The listing builds one solid part. Answer for the finished solid, in the listing's coordinates (mm). Face numbers are marked on the shaded views. A direction names the side the tool comes from. Round coordinates to 2 decimals unless told otherwise and drop trailing zeros. Write each loop counter-clockwise with the first axis right and the second up, starting at its lowest first coordinate (ties: lowest second). Pieces come first, ordered by that corner, then holes. Notation, with made-up numbers: (63.25, 79.5) - (103.25, 79.5) arc R16 cw to (103.25, 88.5) - close; hole circle Ø2 at (-17.5, 76.5). An arc over 180 degrees is marked (long way). Answer in a Markdown table with one row per item.
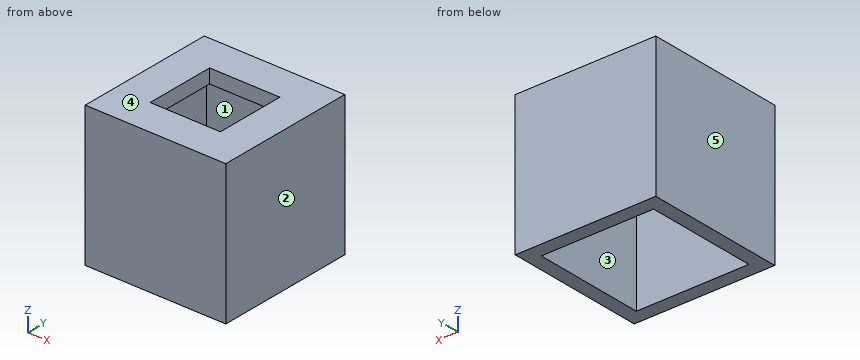
Autodesk Inventor part; units mm, degrees
ref_plane "YZ Plane" through (0, 0, 0) normal (1, 0, 0) x (0, 1, 0)
ref_plane "XZ Plane" through (0, 0, 0) normal (0, 1, 0) x (-1, 0, 0)
ref_plane "XY Plane" through (0, 0, 0) normal (0, 0, 1) x (1, 0, 0)
sketch "Sketch1" plane through (0, 0, 0) normal (0, 0, 1) x (1, 0, 0)
  line L0 (-24.3417, 44.0972) -> (51.8583, 44.0972)
  line L1 (51.8583, 44.0972) -> (51.8583, -32.1028)
  line L2 (51.8583, -32.1028) -> (-24.3417, -32.1028)
  line L3 (-24.3417, -32.1028) -> (-24.3417, 44.0972)
  point P0 (0, 0)
  dimension "d0" = 76.2
  dimension "d1" = 76.2
extrude "Extrusion1" add sketch "Sketch1" along normal blind 76.2
shell "Shell1" thickness 7.62 removed faces 1 at (1.0583, 18.6972, 0)
sketch "Sketch2" plane through (0, 0, 76.2) normal (0, 0, 1) x (1, 0, 0)
  line L0 (-5.2917, 25.0472) -> (32.8083, 25.0472)
  line L1 (32.8083, 25.0472) -> (32.8083, -13.0528)
  line L2 (32.8083, -13.0528) -> (-5.2917, -13.0528)
  line L3 (-5.2917, -13.0528) -> (-5.2917, 25.0472)
  line L4 (51.8583, 44.0972) -> (-24.3417, 44.0972)
  line L5 (51.8583, -32.1028) -> (51.8583, 44.0972)
  point P0 (0, 0)
  dimension "d5" = 38.1
  dimension "d6" = 38.1
  dimension "d7" = 19.05
  dimension "d8" = 19.05
extrude "Extrusion2" cut sketch "Sketch2" against normal blind 25.4
properties part number "secondary_part"
(1) Section C-C (y = 4) is taken. Give the vertices of the cut face in (x, z).
Checked values:
| item | result |
|---|---|
| outline | (-24.34, 0) - (-16.72, 0) - (-16.72, 68.58) - (-5.29, 68.58) - (-5.29, 76.2) - (-24.34, 76.2) - close; (32.81, 68.58) - (44.24, 68.58) - (44.24, 0) - (51.86, 0) - (51.86, 76.2) - (32.81, 76.2) - close |
(2) For the marked faces 1 and 2, determine the directions among +Z, -Z, +X, -X, +Y, -Y from which every point of the face is accessible in a straight line to the end or side of a thin tool.
Checked values:
| item | result |
|---|---|
| face 1 | -Z |
| face 2 | +Z, -Z, +X, +Y, -Y |
(3) Section A-A (z = 23) is taken. Give the vertices of the cut face in (x, y), and give its area (3 significant figures).
Checked values:
| item | result |
|---|---|
| outline | (-24.34, -32.1) - (51.86, -32.1) - (51.86, 44.1) - (-24.34, 44.1) - close; hole (-16.72, -24.48) - (44.24, -24.48) - (44.24, 36.48) - (-16.72, 36.48) - close |
| area | 2,090 mm2 |
(4) For a pull along X with two mould halves and no side action, classify the marked faces 3, 4 and 5 as pulls with the +X half, pulls with the -X half, needs draft (parallel to the pull), parting line crosses it, or undercut.
Checked values:
| item | result |
|---|---|
| face 3 | undercut |
| face 4 | needs draft |
| face 5 | pulls with the -X half |
(5) Section B-B (x = 0) is taken. Give the vertices of the cut face in (y, z).
Checked values:
| item | result |
|---|---|
| outline | (-32.1, 0) - (-24.48, 0) - (-24.48, 68.58) - (-13.05, 68.58) - (-13.05, 76.2) - (-32.1, 76.2) - close; (25.05, 68.58) - (36.48, 68.58) - (36.48, 0) - (44.1, 0) - (44.1, 76.2) - (25.05, 76.2) - close |
(6) Find the intervals of material crossed by line 1 (X direction, y = 15.5, z = 35.5); line 2 (Y direction, x = 22, z = 45); line 3 (Y direction, x = 0, z = 70), in increasing order.
Checked values:
| item | result |
|---|---|
| line 1 | x = -24.34 to -16.72, 44.24 to 51.86 |
| line 2 | y = -32.1 to -24.48, 36.48 to 44.1 |
| line 3 | y = -32.1 to -13.05, 25.05 to 44.1 |
(7) Section D-D (x = 36) is taken. Give the vertices of the cut face in (y, z), and give its area (3 significant figures).
Checked values:
| item | result |
|---|---|
| outline | (-32.1, 0) - (-24.48, 0) - (-24.48, 68.58) - (36.48, 68.58) - (36.48, 0) - (44.1, 0) - (44.1, 76.2) - (-32.1, 76.2) - close |
| area | 1,630 mm2 |
